Solid Edge part; units mm, degrees
sketch "Sketch1" plane through (0, 0, 0) normal (0, -1, 0) x (1, 0, 0)
  line L0 (-7.5, -25) -> (7.5, -25)
  line L1 (7.5, -25) -> (7.5, 25)
  line L2 (7.5, 25) -> (-7.5, 25)
  line L3 (-7.5, 25) -> (-7.5, -25)
  dimension "D1" = 7.5
  dimension "D2" = 7.5
extrude "Protrusion1" add sketch "Sketch1" against normal blind 15
sketch "Sketch2" plane through (7.5, 7.5, 0) normal (1, 0, 0) x (0, 1, 0)
  line L0 (-7.5, 9.5) -> (-7.5, -9.5)
  arc A0 (-7.5, 9.5) -> (-7.5, -9.5) centre (-7.5, 0) cw
extrude "Cutout1" cut sketch "Sketch2" against normal through all
sketch "Sketch3" plane through (0, 0, 0) normal (0, -1, 0) x (1, 0, 0)
  circle A0 centre (0, 15.5) radius 3.25
  circle A1 centre (0, -15.5) radius 3.25
extrude "Cutout2" cut sketch "Sketch3" against normal through all
sketch "Sketch4" plane through (0, 15, 0) normal (0, 1, 0) x (-1, 0, 0)
  circle A0 centre (0, 15.5) radius 7
  circle A1 centre (0, -15.5) radius 7
extrude "ExtrudedCutout_4" cut sketch "Sketch4" against normal blind 8
properties material "Stainless steel"
Input: part model. Units: mm. Frame: model coordinates. A direction names the side the tool comes from. Give positions to 0.01 mm unless a question says otherwise; leave off trailing zeros. Order: outer loops, then holes, each group sorted by start corner. A loop starts at its lowest first (then second) coordinate and runs counter-clockwise, first axis right, second up.
Q1. Draft query along Z for faces 1 (the flat face through (0, 0, 19)), 2 (the cylindrical face through (0.105, 9.498, -0.209)), 3 (the flat face through (0, 7, 25)). Return one class per face: +Z half, -Z half, draft (parallel to the pull), parting line (faces both ways), or undercut.
Checked values:
face 1: draft
face 2: undercut
face 3: +Z half
Q2. Section D-D on y = 13.5. Output: boundary loops of the cut face in (x, z).
Checked values:
outline: (-7.5, -25) - (7.5, -25) - (7.5, 25) - (-7.5, 25) - close; hole circle Ø14 at (0, -15.5); hole circle Ø14 at (0, 15.5)
Q3. Section C-C on y = 8. Output: boundary loops of the cut face in (x, z).
Checked values:
outline: (-7.5, -25) - (7.5, -25) - (7.5, -5.12) - (-7.5, -5.12) - close; (-7.5, 5.12) - (7.5, 5.12) - (7.5, 25) - (-7.5, 25) - close; hole circle Ø14 at (0, -15.5); hole circle Ø14 at (0, 15.5)
Q4. Ray query, probe 1 along Z at (x, y) = (0, 12.75); probe 2 along Z at (x, y) = (0, 5); probe 3 along Z at (x, y) = (5.75, 8.5). Return the intervals inside material, ascending.
Checked values:
probe 1: z = -25 to -22.5, -8.5 to 8.5, 22.5 to 25
probe 2: z = -25 to -18.75, -12.25 to -8.08, 8.08 to 12.25, 18.75 to 25
probe 3: z = -25 to -19.49, -11.51 to -4.24, 4.24 to 11.51, 19.49 to 25
Q5. Contact query for a flat-ended pin moving along its axis: pin 1 Ø7 at (x, z) = (-0.5, -14) entering from +Y. Output: stop coordinate, or through.
Checked values:
pin 1: stops at y = 7
Q6. Section A-A on x = 0. Output: boundary loops of the cut face in (y, z).
Checked values:
outline: (0, -25) - (15, -25) - (15, -22.5) - (7, -22.5) - (7, -18.75) - (0, -18.75) - close; (0, -12.25) - (7, -12.25) - (7, -8.5) - (15, -8.5) - (15, 8.5) - (7, 8.5) - (7, 12.25) - (0, 12.25) - (0, 9.5) arc R9.5 cw to (0, -9.5) - close; (0, 18.75) - (7, 18.75) - (7, 22.5) - (15, 22.5) - (15, 25) - (0, 25) - close
Q7. Set-up query: faces 4 (the flat face through (-1, 7, -12)), 5 (the cylindrical face through (-0.423, 3.451, 18.722)). Return all of +Z, -Z, +X, -X, +Y, -Y with unobstructed straight access to the full face (end or side cutting, diameter ignored); none if empty.
Checked values:
face 4: +Y
face 5: +Y, -Y
Q8. Section B-B on z = -15.5. Output: boundary loops of the cut face in (x, y).
Checked values:
outline: (-7.5, 0) - (-3.25, 0) - (-3.25, 7) - (-7, 7) - (-7, 15) - (-7.5, 15) - close; (3.25, 0) - (7.5, 0) - (7.5, 15) - (7, 15) - (7, 7) - (3.25, 7) - close
